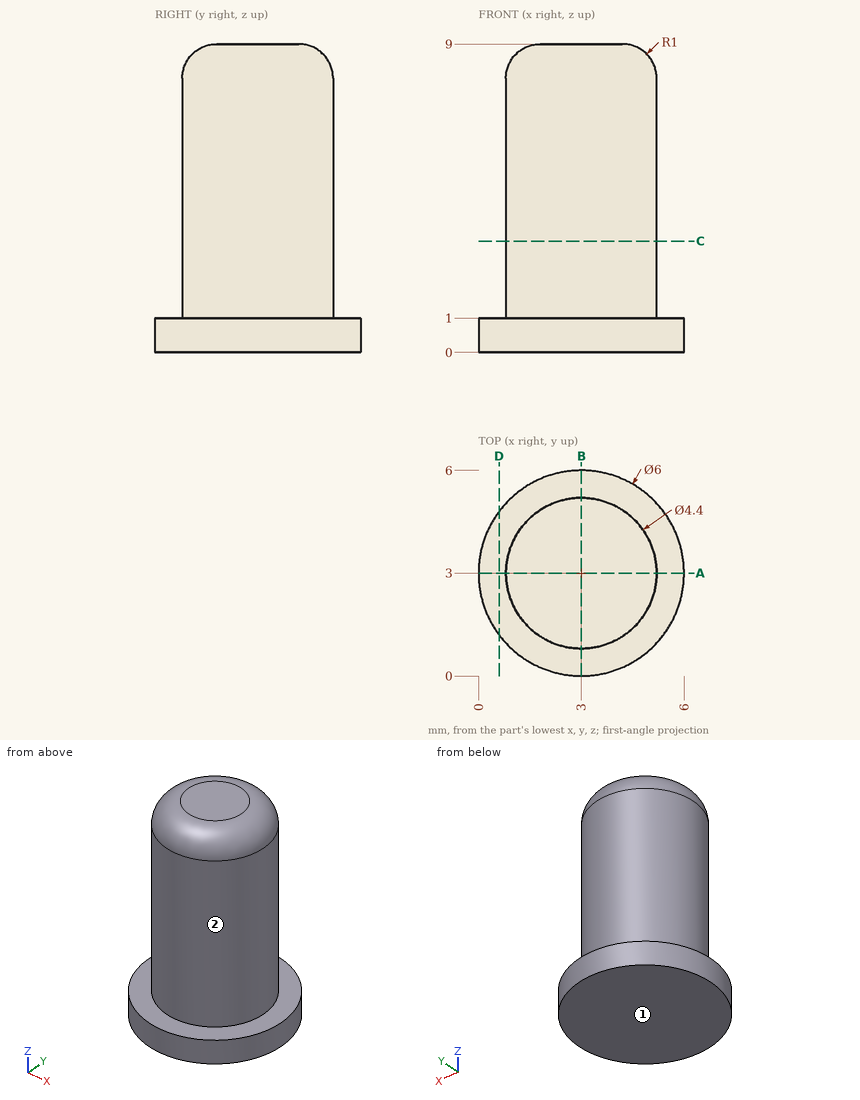
Source: three-view drawing plus pictorial views. Frame: mm from the lowest corner of the part. A direction names the side the tool comes from. Give positions to 0.01 mm unless a question says otherwise; leave off trailing zeros. Order: outer loops, then holes, each group sorted by start corner. A loop starts at its lowest first (then second) coordinate and runs counter-clockwise, first axis right, second up. Notation, with made-up numbers: M -25,41.25 L -19,41.25 A25 ccw -19,76.25 Z; hole C 29,53.25 d10. An arc over 180 degrees is marked long. One line per question, with ' | ' between items.
1) Access query for the marked faces 1 and 2. Directions: +Z, -Z, +X, -X, +Y, -Y. A direction counts if a zero-diameter tool reaches every point of the face in a straight line with its end or side. Return the directions, or none.
Filled in:
face 1: -Z, +X, -X, +Y, -Y | face 2: +Z
2) Contact query for flat-ended pins moving along their axis: P1, Ø1.5, axis at y = 3.5, z = 6, coming from the -X side; P2, Ø1.5, axis at y = 5, z = 2.5, coming from the -X side. Output: stop coordinate, or through.
Filled in:
P1: stops at x = 0.8 | P2: stops at x = 1.19
3) Section C-C on z = 3.25. Output: boundary loops of the cut face in (x, y).
Filled in:
outline: C 3,3 d4.4
4) Section D-D on x = 0.6. Output: boundary loops of the cut face in (y, z).
Filled in:
outline: M 1.2,0 L 4.8,0 L 4.8,1 L 1.2,1 Z
5) Section A-A on y = 3. Output: boundary loops of the cut face in (x, z).
Filled in:
outline: M 0,0 L 6,0 L 6,1 L 5.2,1 L 5.2,8 A1 ccw 4.2,9 L 1.8,9 A1 ccw 0.8,8 L 0.8,1 L 0,1 Z
6) Ray query, L1, parallel to Z at x = 1.25, y = 4.7; L2, parallel to X at y = 2.95, z = 2.5; L3, parallel to Y at x = 4, z = 4.5. Return the intervals inside material, ascending.
Filled in:
L1: z = 0 to 1 | L2: x = 0.8 to 5.2 | L3: y = 1.04 to 4.96
